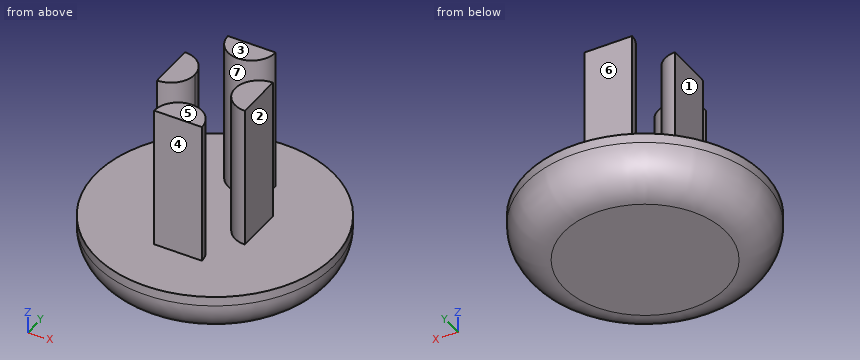
```python
from build123d import *

# Parameters (mm, degrees)
F0_R     = 12.5
F1_DEPTH = 5
F2_R     = 4
F4_DEPTH = 15


with BuildPart() as f1:
    # F0 (on Top) → F1 (new body)
    with BuildSketch(Plane.XY):
        Circle(F0_R)
    extrude(amount=F1_DEPTH)

    # F2
    f2_edges = [f1.edges().sort_by_distance(p)[0] for p in [
        (-12.5, 0, 0),
    ]]
    fillet(f2_edges, radius=F2_R)

    # F3 (on face) → F4 (join)
    with BuildSketch(Plane.XY.offset(5)):
        with BuildLine():
            Line((-2.5, -6.6), (2.5, -6.6))
            ThreePointArc((2.5, -6.6), (0, -4.1), (-2.5, -6.6))
        make_face()
        with BuildLine():
            ThreePointArc((-2.5, 6.6), (0, 4.1), (2.5, 6.6))
            Line((2.5, 6.6), (-2.5, 6.6))
        make_face()
        with BuildLine():
            ThreePointArc((4.6, 2.5), (2.1, 0), (4.6, -2.5))
            Line((4.6, -2.5), (4.6, 2.5))
        make_face()
        with BuildLine():
            Line((-4.6, 2.5), (-4.6, -2.5))
            ThreePointArc((-4.6, -2.5), (-2.832233047, -1.767766953), (-2.1, 0))
            ThreePointArc((-2.1, 0), (-2.832233047, 1.767766953), (-4.6, 2.5))
        make_face()
    extrude(amount=F4_DEPTH)


solid = f1.part
```
The model under review builds one solid part; all positions refer to its coordinate system, in mm. Face numbers are marked on the shaded views. A direction names the side the tool comes from. Round coordinates to 2 decimals unless told otherwise and drop trailing zeros. Write each loop counter-clockwise with the first axis right and the second up, starting at its lowest first coordinate (ties: lowest second). Pieces come first, ordered by that corner, then holes.
(1) Wall thickness on L1, parallel to Y at x = 0, z = 8; L2, parallel to Z at x = -2.5, y = -4.75; L3, parallel to X at y = 0.5, z = 18.5: over which ranges is each line inside the solid? List them lowest first.
(2) Machinability: for the marked faces 1, 2 and 3, which of the approach directions +Z, -Z, +X, -X, +Y, -Y give a long, thin tool a straight path to every point of the face, cutting with its end or side? Answer none if there is none.
(3) We need section B-B on x = 0. Give the boundary of the cut face in (y, z), and give its area (3 significant figures).
(4) We need section A-A on z = 11.75. Give the boundary of the cut face in (x, y), and give its area (3 significant figures).
(5) Mouldability with a two-part tool opening along Y and no side actions: class the marked faces 4, 5, 6 and 7 as +Y half, -Y half, draft (parallel to the pull), parting line (faces both ways), or undercut.
(6) We need section C-C on z = 1.25. Give the boundary of the cut face in (x, y).
(7) Insertion check: pin 1 (4 mm diameter, centred on x = -4, z = 8, fed in from -Y); pin 2 (4 mm diameter, centred on y = -8, z = 12.5, fed in from +X); pin 3 (12 mm diameter, centred on y = -4.5, z = 9, fed in from +X). Each pin has a flat end and moves straight along its axis. Give the tip position at first contact, or say it passes through.
Findings below:
1. L1: y = -6.6 to -4.1, 4.1 to 6.6
1. L2: z = 0 to 5
1. L3: x = -4.6 to -2.15, 2.15 to 4.6
2. face 1: +Z, -X, +Y, -Y
2. face 2: +Z, +X, +Y, -Y
2. face 3: +Z, +X, -X, +Y, -Y
3. outline: (-12.5, 4) arc R4 ccw to (-8.5, 0) - (8.5, 0) arc R4 ccw to (12.5, 4) - (12.5, 5) - (6.6, 5) - (6.6, 20) - (4.1, 20) - (4.1, 5) - (-4.1, 5) - (-4.1, 20) - (-6.6, 20) - (-6.6, 5) - (-12.5, 5) - close
3. area: 193 mm2
4. outline: (-4.6, -2.5) arc R2.5 ccw to (-4.6, 2.5) - close; (-2.5, -6.6) - (2.5, -6.6) arc R2.5 ccw to start; (-2.5, 6.6) arc R2.5 ccw to (2.5, 6.6) - close; (4.6, -2.5) - (4.6, 2.5) arc R2.5 ccw to start
4. area: 39.3 mm2
5. face 4: -Y half
5. face 5: draft
5. face 6: +Y half
5. face 7: undercut
6. outline: circle Ø22.81 at (0, 0)
7. pin 1: stops at y = -6.6
7. pin 2: stops at x = 2.5
7. pin 3: stops at x = 12.5
